Read the model definition and answer for the solid it produces. Units are mm, in the model's axes. Coordinates: 2 decimals unless noted, no trailing zeros. Write each loop counter-clockwise with the first axis right and the second up, starting at its lowest first coordinate (ties: lowest second). Pieces come first, ordered by that corner, then holes. Notation, with made-up numbers: (-33, 34.5) -> (-28, 34.5) arc R7 cw to (-28, 41.5) -> close; hole circle Ø9 at (33, 70). An arc over 180 degrees is marked (long way). Write item = value, one per line. Start each with the question number.
1) Section D-D (x = 2.4) is taken. Count the separate pieces of the cut face and the enclosed holes in it, plus the area to 3 significant figures.
2) Find the intervals of material crossed by line 1 along Z through (x, y) = (0.7, 38); line 2 along Y through (x, z) = (0.5, -28); line 3 along Y through (x, z) = (0.8, -37), in increasing order. Write a range as from..to.
3) Section C-C (y = 12.5) is taken. Determine the outline of the cut face in (x, z).
4) Flat-ended cylindrical pins translate along their axes: pin 1 Ø1 at (y, z) = (26.5, -32) entering from +X; pin 2 Ø1.3 at (x, z) = (2, -9) entering from +Y. Find the tip coordinate at first contact, or state that the pin passes through.
5) Section B-B (y = 21.25) is taken. Determine the outline of the cut face in (x, z), plus the area to 3 significant figures.
6) Section A-A (y = 29) is taken. Determine the outline of the cut face in (x, z).
Autodesk Inventor part; units mm, degrees
ref_plane "YZ Plane" through (0, 0, 0) normal (1, 0, 0) x (0, 1, 0)
ref_plane "XZ Plane" through (0, 0, 0) normal (0, 1, 0) x (-1, 0, 0)
ref_plane "XY Plane" through (0, 0, 0) normal (0, 0, 1) x (1, 0, 0)
sketch "Sketch1" plane through (0, 0, 0) normal (1, 0, 0) x (0, 1, 0)
  line L0 (0, 0) -> (45, 0)
  line L1 (45, 0) -> (45, -42)
  line L2 (45, -42) -> (0, -42)
  line L3 (0, -42) -> (0, 0)
  dimension "d0" = 45
  dimension "d1" = 42
extrude "Extrusion1" add sketch "Sketch1" along normal blind 3
sketch "Sketch4" plane through (0, 0, 0) normal (-1, 0, 0) x (0, 0, 1)
  circle A0 centre (-2.5714, 12) radius 1.5
  circle A1 centre (-36.5714, 21.25) radius 1.5
  circle A2 centre (-36.5714, 3.75) radius 1.5
  circle A3 centre (-16.9627, 12.5) radius 5
  line L0 (-42, 0) -> (0, 0)
  circle A4 centre (-27.9627, 12.5) radius 2
  point P0 (0, 10)
  point P1 (-32, 0)
  point P2 (-10, 0)
  dimension "d21" = 3
  dimension "d23" = 3
  dimension "d26" = 3
  dimension "d29" = 10
  dimension "d32" = 12.5
  dimension "d76" = 4
  dimension "d77" = 4
  dimension "d78" = 12.5
  dimension "d79" = 7.9
extrude "Extrusion4" cut sketch "Sketch4" against normal blind 4
sketch "Sketch5" plane through (0, 0, 0) normal (-1, 0, 0) x (0, 0, 1)
  line L0 (-16, 45) -> (-16, 42)
  line L1 (-26, 42) -> (-26, 45)
  line L2 (-36, 45) -> (-36, 42)
  line L3 (-42, 42) -> (-42, 45)
  line L4 (-6, 45) -> (-6, 42)
  line L5 (-42, 45) -> (0, 45)
  line L6 (-6, 45) -> (-16, 45)
  line L7 (-16, 42) -> (-16, 45)
  line L8 (-26, 45) -> (-36, 45)
  line L9 (-9.4, 24.8) -> (-12.6, 24.8)
  line L10 (-9.4, 34.2) -> (-8.2, 34.2)
  line L11 (-8.2, 34.2) -> (-8.2, 31.45)
  line L12 (-8.2, 31.45) -> (-9.4, 31.45)
  line L13 (-12.6, 34.2) -> (-13.8, 34.2)
  line L14 (-13.8, 34.2) -> (-13.8, 31.45)
  line L15 (-12.6, 31.45) -> (-13.8, 31.45)
  line L16 (-9.4, 42) -> (-9.4, 34.2)
  line L17 (-9.4, 31.45) -> (-9.4, 24.8)
  line L18 (-12.6, 24.8) -> (-12.6, 31.45)
  line L19 (-12.6, 34.2) -> (-12.6, 42)
  line L20 (-6, 42) -> (-9.4, 42)
  line L21 (-12.6, 42) -> (-16, 42)
  line L22 (-26, 42) -> (-29.4, 42)
  line L23 (-29.4, 42) -> (-29.4, 34.2)
  line L24 (-29.4, 34.2) -> (-28.2, 34.2)
  line L25 (-28.2, 34.2) -> (-28.2, 31.45)
  line L26 (-28.2, 31.45) -> (-29.4, 31.45)
  line L27 (-29.4, 31.45) -> (-29.4, 24.8)
  line L28 (-29.4, 24.8) -> (-32.6, 24.8)
  line L29 (-32.6, 24.8) -> (-32.6, 31.45)
  line L30 (-32.6, 31.45) -> (-33.8, 31.45)
  line L31 (-33.8, 31.45) -> (-33.8, 34.2)
  line L32 (-33.8, 34.2) -> (-32.6, 34.2)
  line L33 (-32.6, 34.2) -> (-32.6, 42)
  line L34 (-32.6, 42) -> (-36, 42)
  dimension "d38" = 10
  dimension "d42" = 6
  dimension "d47" = 10
  dimension "d48" = 10
  dimension "d55" = 2.75
  dimension "d59" = 3
  dimension "d60" = 7.8
  dimension "d61" = 6.65
  dimension "d62" = 5.6
  dimension "d63" = 3.2
  dimension "d64" = 3.4
  dimension "d65" = 3.4
  dimension "d66" = 7.8
  dimension "d67" = 1.2
  dimension "d68" = 1.2
  dimension "d69" = 2.75
  dimension "d70" = 3.2
  dimension "d71" = 1.2
  dimension "d72" = 1.2
  dimension "d73" = 6.65
  dimension "d74" = 7.8
  dimension "d75" = 20.2
extrude "Extrusion5" cut sketch "Sketch5" against normal blind 4
fillet "Fillet2" radius 7 2 edges at (1.5, 0, 0) (1.5, 0, -42)
properties part number "motor mount" material "Plywood, Finish"
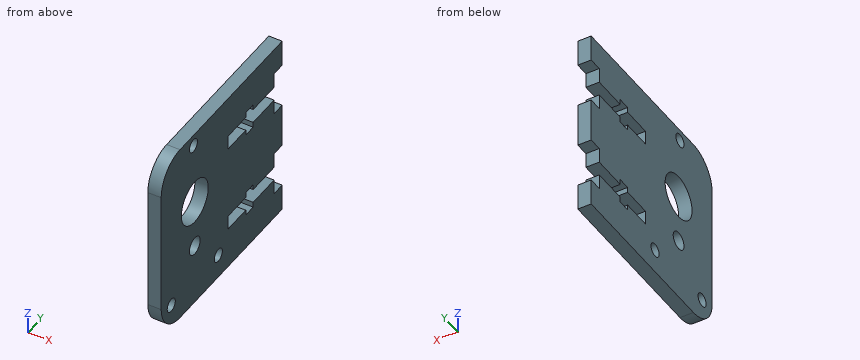
Answer key:
q1.separate_pieces = 1
q1.enclosed_holes = 5
q1.area = 1,570 mm^2
q2.line_1 = -42..-32.6, -29.4..-12.6, -9.4..0
q2.line_2 = 0..10.5, 14.5..42
q2.line_3 = 0.29..2.31, 5.19..19.81, 22.69..45
q3.outline = (0, -42) -> (3, -42) -> (3, -29.96) -> (0, -29.96) -> close; (0, -25.96) -> (3, -25.96) -> (3, -21.96) -> (0, -21.96) -> close; (0, -11.96) -> (3, -11.96) -> (3, -3.99) -> (0, -3.99) -> close; (0, -1.16) -> (3, -1.16) -> (3, 0) -> (0, 0) -> close
q4.pin_1 = through
q4.pin_2 = 42
q5.outline = (0, -42) -> (3, -42) -> (3, -38.07) -> (0, -38.07) -> close; (0, -35.07) -> (3, -35.07) -> (3, 0) -> (0, 0) -> close
q5.area = 117 mm^2
q6.outline = (0, -42) -> (3, -42) -> (3, -32.6) -> (0, -32.6) -> close; (0, -29.4) -> (3, -29.4) -> (3, -12.6) -> (0, -12.6) -> close; (0, -9.4) -> (3, -9.4) -> (3, 0) -> (0, 0) -> close
